Geometry: see drawing. Coordinates: mm, zero at the bounding-box minimum. Coordinates: 2 decimals unless noted, no trailing zeros. Order: outer loops, then holes, each group sorted by start corner. A loop starts at its lowest first (then second) coordinate and runs counter-clockwise, first axis right, second up. Notation, with made-up numbers: (88, 56.5) -> (103, 56.5) arc R19 cw to (103, 65.5) -> close; hole circle Ø9 at (81, 66.5). An arc over 180 degrees is marked (long way). Use CSV: the item, a comma, the result in double quotes. Start each with the question number.
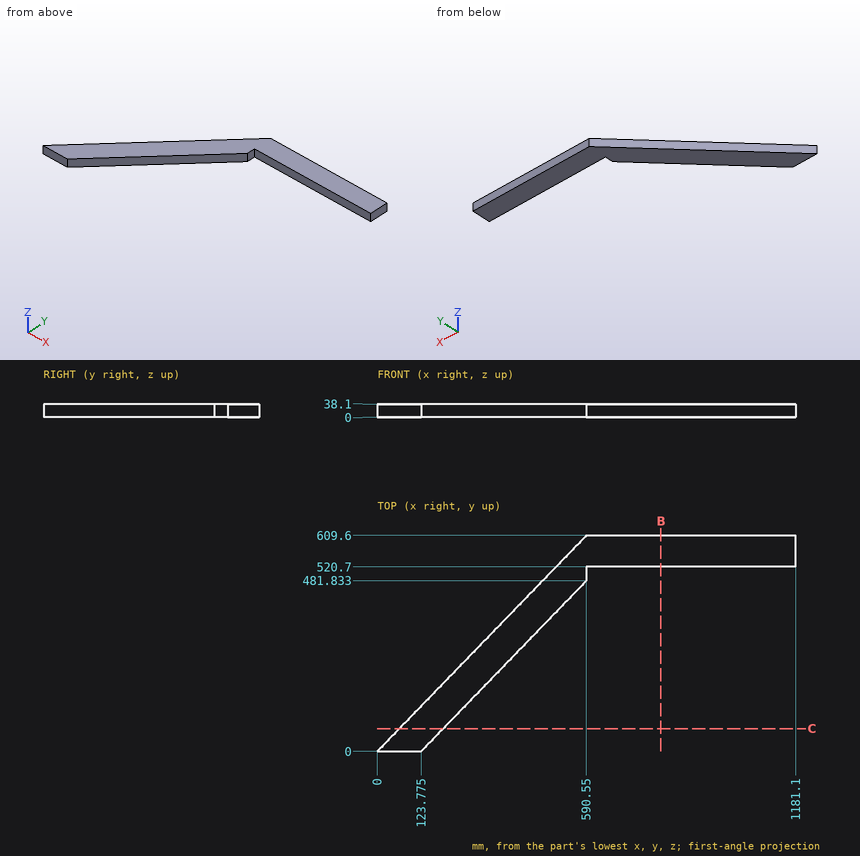
(1) Line query: line 1 (Y direction, x = 618, z = 31); line 2 (X direction, y = 389.5, z = 26.5) (1 decimal); line 3 (X direction, y = 224, z = 31.5) (1 decimal). Output: solid intervals per line, ascending. Write a range as from..to.
(2) First-contact query: pin 1 (5 mm diameter, centred on y = 494, z = 22, fed in from +X); pin 2 (1 mm diameter, centred on y = 356, z = 5.5, fed in from +X) (1 decimal); pin 3 (8 mm diameter, centred on x = 426, z = 19, fed in from -Y) (1 decimal). Flat tips, straight axial feed; report the tip coordinate or a pass-through.
(3) Section B-B (x = 800.5). Return loops of the section in (y, z), then the cut area to 3 significant figures.
(4) Section C-C (y = 64). Return loops of the section in (x, z) (1 decimal).
Check sheet entries:
1,line 1,"y = 520.7..609.6"
1,line 2,"x = 377.3..501.1"
1,line 3,"x = 217..340.8"
2,pin 1,"stops at x = 590.55"
2,pin 2,"stops at x = 469.1"
2,pin 3,"stops at y = 307.8"
3,outline,"(520.7, 0) -> (609.6, 0) -> (609.6, 38.1) -> (520.7, 38.1) -> close"
3,area,"3,390 mm^2"
4,outline,"(62, 0) -> (185.8, 0) -> (185.8, 38.1) -> (62, 38.1) -> close"
